from build123d import *

# Parameters (mm, degrees)
SKETCH_1_W          = 100
SKETCH_1_H          = 100
EXTRUDE_1_DEPTH     = 2
SKETCH_3_R          = 1.5
CUT_EXTRUDE_2_DEPTH = 71.738956735
SKETCH_4_R          = 1.5
CUT_EXTRUDE_3_DEPTH = 71.738956735
SKETCH_5_W          = 2
SKETCH_5_H          = 40
CUT_EXTRUDE_4_DEPTH = 71.738956735


with BuildPart() as part:
    # 草图1 → 凸台-拉伸1 (new body)
    with BuildSketch(Plane(origin=(0, 0, 0), x_dir=(1, 0, 0), z_dir=(0, 1, 0))):
        Rectangle(SKETCH_1_W, SKETCH_1_H)
    extrude(amount=EXTRUDE_1_DEPTH)

    # 草图3 → 切除-拉伸2 (cut, through all)
    with BuildSketch(Plane(origin=(0, 2, 0), x_dir=(1, 0, 0), z_dir=(0, 1, 0))):
        with Locations(Location((-42.426406871, 42.426406871, 0), (0, 0, 270))):
            Circle(SKETCH_3_R)
        with Locations(Location((-31.819805153, 38.890872965, 0), (0, 0, 270))):
            Circle(SKETCH_3_R)
        with Locations(Location((-38.890872965, 31.819805153, 0), (0, 0, 270))):
            Circle(SKETCH_3_R)
        with Locations(Location((-31.819805153, -38.890872965, 0), (0, 0, 90))):
            Circle(SKETCH_3_R)
        with Locations(Location((-38.890872965, -31.819805153, 0), (0, 0, 90))):
            Circle(SKETCH_3_R)
        with Locations(Location((-42.426406871, -42.426406871, 0), (0, 0, 90))):
            Circle(SKETCH_3_R)
        with Locations(Location((31.819805153, 38.890872965, 0), (0, 0, 90))):
            Circle(SKETCH_3_R)
        with Locations(Location((38.890872965, 31.819805153, 0), (0, 0, 90))):
            Circle(SKETCH_3_R)
        with Locations(Location((42.426406871, 42.426406871, 0), (0, 0, 90))):
            Circle(SKETCH_3_R)
        with Locations(Location((31.819805153, -38.890872965, 0), (0, 0, 270))):
            Circle(SKETCH_3_R)
        with Locations(Location((42.426406871, -42.426406871, 0), (0, 0, 270))):
            Circle(SKETCH_3_R)
        with Locations(Location((38.890872965, -31.819805153, 0), (0, 0, 270))):
            Circle(SKETCH_3_R)
    extrude(amount=-CUT_EXTRUDE_2_DEPTH, mode=Mode.SUBTRACT)

    # 草图4 → 切除-拉伸3 (cut, through all)
    with BuildSketch(Plane.XZ):
        with Locations(Location((-39.5, 21, 0), (0, 0, 270))):
            Circle(SKETCH_4_R)
        with Locations(Location((39.5, 21, 0), (0, 0, 90))):
            Circle(SKETCH_4_R)
        with Locations(Location((39.5, -21, 0), (0, 0, 270))):
            Circle(SKETCH_4_R)
        with Locations(Location((-39.5, -21, 0), (0, 0, 90))):
            Circle(SKETCH_4_R)
    extrude(amount=-CUT_EXTRUDE_3_DEPTH, mode=Mode.SUBTRACT)

    # 草图5 → 切除-拉伸4 (cut, through all)
    with BuildSketch(Plane.XZ):
        with Locations((-46, 0)):
            Rectangle(SKETCH_5_W, SKETCH_5_H)
        with Locations((46, 0)):
            Rectangle(SKETCH_5_W, SKETCH_5_H)
    extrude(amount=-CUT_EXTRUDE_4_DEPTH, mode=Mode.SUBTRACT)


solid = part.part
Geometry check sheet. Reference: the model listing, model coordinates, mm. Round coordinates to 2 decimals unless told otherwise and drop trailing zeros. Order: outer loops, then holes, each group sorted by start corner. A loop starts at its lowest first (then second) coordinate and runs counter-clockwise, first axis right, second up. Notation, with made-up numbers: M 3,86.5 L 41,86.5 A32 ccw 41,115.5 Z; hole C 34.5,54.25 d5. An arc over 180 degrees is marked long. Answer in a Markdown table with one row per item. Add a question column.
Item 1: Material ranges on L1, parallel to X at y = 0.75, z = 3; L2, parallel to X at y = 1.65, z = -33; L3, parallel to Z at x = -39, y = 0.9, recorded low to high. Write a range as [from, to].
Item 2: Draft check along X on faces 1 (the face through (-1, 0, -1)), 2 (the face through (30.5, 1, 39.6)). Enter one of: released by +X, released by -X, zero draft, split by the parting line, or undercut.
Item 3: Sectioned sample at B-B, the plane y = 1.6. State how many separate pieces and enclosed holes the cut face has, plus the area to 3 significant figures.
Item 4: Sectioned sample at A-A, the plane z = 18. Enter the section's corners in (x, y).
Filled in:
| question | item | result |
|---|---|---|
| 1 | L1 | x = [-50, -47], [-45, 45], [47, 50] |
| 1 | L2 | x = [-50, -39.82], [-37.97, 37.97], [39.82, 50] |
| 1 | L3 | z = [-50, -33.32], [-30.32, -22.41], [-19.59, 19.59], [22.41, 30.32], [33.32, 50] |
| 2 | face 1 | zero draft |
| 2 | face 2 | undercut |
| 3 | separate pieces | 1 |
| 3 | enclosed holes | 18 |
| 3 | area | 9,730 mm² |
| 4 | outline | M -50,0 L -47,0 L -47,2 L -50,2 Z; M -45,0 L 45,0 L 45,2 L -45,2 Z; M 47,0 L 50,0 L 50,2 L 47,2 Z |
